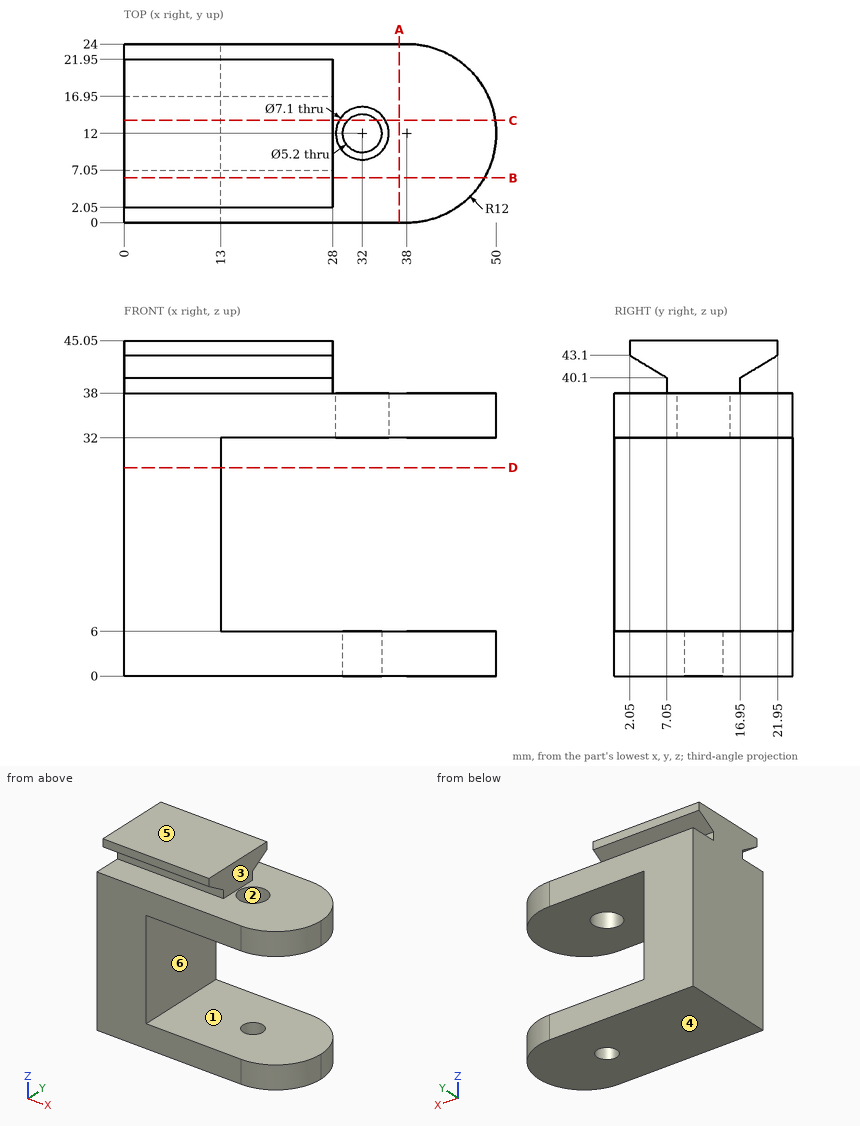
Can you work these out from the drawing? Everything is in mm from the part's minimum corner. A direction names the side the tool comes from. Round coordinates to 2 decimals unless told otherwise and drop trailing zeros. Write each loop counter-clockwise with the first axis right and the second up, starting at its lowest first coordinate (ties: lowest second). Pieces come first, ordered by that corner, then holes. Notation, with made-up numbers: (27, 85) - (84, 85) arc R23 cw to (84, 123) - close; hole circle Ø5 at (57, -25.75). An arc over 180 degrees is marked (long way). Write each question's results on one line, items separated by ' | '. Start each with the question number.
1) Suppose I cut it at D-D (z = 28). List the corners of the cut face in (x, y) for me.
2) Suppose I cut it at A-A (x = 37). List the corners of the cut face in (y, z) for me.
3) Which directions (+Z, -Z, +X, -X, +Y, -Y) give clear straight access to the entire face, cutting with the end or side of a thin tool? Please do the marked faces 1, 2 and 3.
4) For pin 1 Ø2 at (y, z) = (12, 40.5) entering from +X; pin 2 Ø2 at (x, z) = (8, 44) entering from +Y; pin 3 Ø10 at (y, z) = (4, 31) entering from +X, each with a flat end and sliding along its axis, tell me the tip position at first contact or that it passes through.
5) Please list where these lines run through material, in increasing order: line 1 (Y direction, x = 32, z = 2.75); line 2 (Z direction, x = 40, y = 7.5); line 3 (Y direction, x = 32, z = 36.5).
6) We'd pull the mould along Z, two halves only. Please class the marked faces 4, 5 and 6: released by +Z, released by -Z, zero draft, split by the parting line, or undercut.
7) Suppose I cut it at C-C (y = 13.75). List the corners of the cut face in (x, z) for me.
8) Suppose I cut it at B-B (y = 6). List the corners of the cut face in (x, z) for me, and give its area (3 significant figures).
Here are the results:
1) outline: (0, 0) - (13, 0) - (13, 24) - (0, 24) - close
2) outline: (0, 0) - (24, 0) - (24, 6) - (0, 6) - close; (0, 32) - (24, 32) - (24, 38) - (0, 38) - close
3) face 1: +X, +Y, -Y | face 2: +Z | face 3: +Z, +X, +Y, -Y
4) pin 1: stops at x = 28 | pin 2: stops at y = 21.95 | pin 3: stops at x = 49.59
5) line 1: y = 0 to 9.4, 14.6 to 24 | line 2: z = 0 to 6, 32 to 38 | line 3: y = 0 to 8.45, 15.55 to 24
6) face 4: released by -Z | face 5: released by +Z | face 6: undercut
7) outline: (0, 0) - (30.08, 0) - (30.08, 6) - (13, 6) - (13, 32) - (28.91, 32) - (28.91, 38) - (28, 38) - (28, 45.05) - (0, 45.05) - close; (33.92, 0) - (49.87, 0) - (49.87, 6) - (33.92, 6) - close; (35.09, 32) - (49.87, 32) - (49.87, 38) - (35.09, 38) - close
8) outline: (0, 0) - (48.39, 0) - (48.39, 6) - (13, 6) - (13, 32) - (48.39, 32) - (48.39, 38) - (0, 38) - close; (0, 40.73) - (28, 40.73) - (28, 45.05) - (0, 45.05) - close | area: 1,040 mm2
